Model file for the job. Use its own axes, mm. Face numbers are marked on the shaded views. A direction names the side the tool comes from. Give positions to 0.01 mm unless a question says otherwise; leave off trailing zeros. Write each loop counter-clockwise with the first axis right and the second up, starting at its lowest first coordinate (ties: lowest second). Pieces come first, ordered by that corner, then holes.
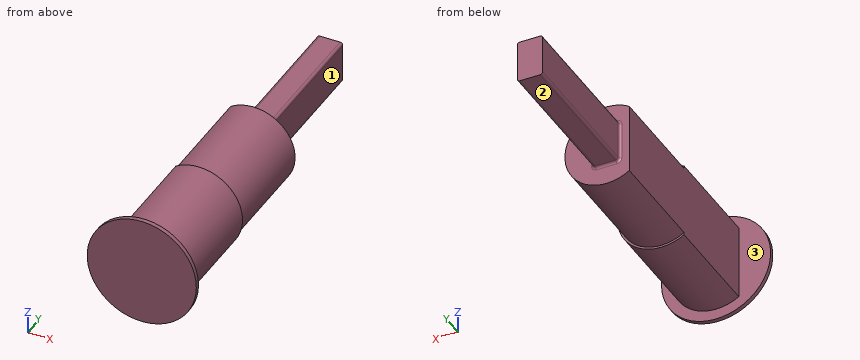
```python
from build123d import *

# Parameters (mm, degrees)
BOSS_EXTRUDE1_DEPTH = 25.4
BOSS_EXTRUDE2_DEPTH = 17.78
FILLET1_R           = 0.3
SKETCH3_R           = 6.46557
BOSS_EXTRUDE3_DEPTH = 0.508
SKETCH4_OUTSIDE_W   = 24.404
SKETCH4_OUTSIDE_H   = 24.404
SKETCH4_OUTSIDE_R   = 4.94157
CUT_EXTRUDE1_DEPTH  = 12.7


with BuildPart() as part:
    # Sketch1 → Boss-Extrude1 (new body)
    with BuildSketch(Plane(origin=(0, 0, 0), x_dir=(1, 0, 0), z_dir=(0, 1, 0))):
        with BuildLine():
            Line((-2.68996703, 4.445), (-2.68996703, -4.445))
            ThreePointArc((-2.68996703, -4.445), (5.19557, 0), (-2.68996703, 4.445))
        make_face()
    extrude(amount=BOSS_EXTRUDE1_DEPTH)

    # Sketch2 → Boss-Extrude2 (add)
    with BuildSketch(Plane(origin=(0, 25.4, 0), x_dir=(1, 0, 0), z_dir=(0, 1, 0))):
        with BuildLine():
            Line((-1.2, -2.5), (1.2, -2.5))
            ThreePointArc((1.2, -2.5), (1.412132034, -2.412132034), (1.5, -2.2))
            Line((1.5, -2.2), (1.5, 2.2))
            ThreePointArc((1.5, 2.2), (1.412132034, 2.412132034), (1.2, 2.5))
            Line((1.2, 2.5), (-1.2, 2.5))
            ThreePointArc((-1.2, 2.5), (-1.412132034, 2.412132034), (-1.5, 2.2))
            Line((-1.5, 2.2), (-1.5, -2.2))
            ThreePointArc((-1.5, -2.2), (-1.412132034, -2.412132034), (-1.2, -2.5))
        make_face()
    extrude(amount=BOSS_EXTRUDE2_DEPTH)

    # Fillet1
    fillet1_edges = [part.edges().sort_by_distance(p)[0] for p in [
        (-1.412132034, 25.4, 2.412132034),
        (0, 25.4, 2.5),
        (1.412132034, 25.4, 2.412132034),
        (1.5, 25.4, 0),
        (1.412132034, 25.4, -2.412132034),
        (0, 25.4, -2.5),
        (-1.412132034, 25.4, -2.412132034),
        (-1.5, 25.4, 0),
    ]]
    fillet(fillet1_edges, radius=FILLET1_R)

    # Sketch3 → Boss-Extrude3 (add)
    with BuildSketch(Plane.XZ):
        Circle(SKETCH3_R)
    extrude(amount=BOSS_EXTRUDE3_DEPTH)

    # Sketch4 outside → Cut-Extrude1 (cut)
    with BuildSketch(Plane(origin=(0, 25.4, 0), x_dir=(1, 0, 0), z_dir=(0, 1, 0))):
        Rectangle(SKETCH4_OUTSIDE_W, SKETCH4_OUTSIDE_H)
        Circle(SKETCH4_OUTSIDE_R, mode=Mode.SUBTRACT)
    extrude(amount=-CUT_EXTRUDE1_DEPTH, mode=Mode.SUBTRACT)


solid = part.part
```
1. Pin check, flat tips, straight feed: P1, Ø1.5, axis at y = 8, z = -3.5, coming from the -X side; P2, Ø2.5, axis at x = 0.5, y = 31.5, coming from the -Z side; P3, Ø1.2, axis at x = 0.5, y = 38.5, coming from the +Z side. Stop position of each tip, or through.
Calculated:
P1: stops at x = -2.69
P2: stops at z = -2.5
P3: stops at z = 2.5
2. Slice it at B-B, the plane y = 28.5. Write the cut outline in (x, z).
Calculated:
outline: (-1.5, -2.2) arc R0.3 ccw to (-1.2, -2.5) - (1.2, -2.5) arc R0.3 ccw to (1.5, -2.2) - (1.5, 2.2) arc R0.3 ccw to (1.2, 2.5) - (-1.2, 2.5) arc R0.3 ccw to (-1.5, 2.2) - close
3. Which spindle directions (+Z, -Z, +X, -X, +Y, -Y) get a long thin tool onto all of the face, cutting with end or side? Do the marked faces 1, 2 and 3. Say none if no direction does.
Calculated:
face 1: +Z, -Z, +X, +Y
face 2: -Z, +X, -X, +Y
face 3: +Y
4. Probe probe 1 along Y at (x, z) = (2.5, 0.75); probe 2 along Y at (x, z) = (0.5, 5.25); probe 3 along Z at (x, y) = (1.25, 35). List the from-to ranges inside material, lowest first.
Calculated:
probe 1: y = -0.51 to 25.4
probe 2: y = -0.51 to 0
probe 3: z = -2.5 to 2.5
5. Slice it at A-A, the plane x = 0. Write the cut outline in (y, z).
Calculated:
outline: (-0.51, -6.47) - (0, -6.47) - (0, -5.2) - (12.7, -5.2) - (12.7, -4.94) - (25.4, -4.94) - (25.4, -2.8) arc R0.3 cw to (25.7, -2.5) - (43.18, -2.5) - (43.18, 2.5) - (25.7, 2.5) arc R0.3 cw to (25.4, 2.8) - (25.4, 4.94) - (12.7, 4.94) - (12.7, 5.2) - (0, 5.2) - (0, 6.47) - (-0.51, 6.47) - close
6. Slice it at C-C, the plane z = 0. Write the cut outline in (x, y).
Calculated:
outline: (-6.47, -0.51) - (6.47, -0.51) - (6.47, 0) - (5.2, 0) - (5.2, 12.7) - (4.94, 12.7) - (4.94, 25.4) - (1.8, 25.4) arc R0.3 cw to (1.5, 25.7) - (1.5, 43.18) - (-1.5, 43.18) - (-1.5, 25.7) arc R0.3 cw to (-1.8, 25.4) - (-2.69, 25.4) - (-2.69, 0) - (-6.47, 0) - close
7. Slice it at D-D, the plane y = 11.5. Write the cut outline in (x, z) (3 decimals).
Calculated:
outline: (-2.69, -4.445) arc R5.196 ccw (long way) to (-2.69, 4.445) - close
